Verification items for the finished model (mm, model axes). A direction names the side the tool comes from. Round coordinates to 2 decimals unless told otherwise and drop trailing zeros. Loops run counter-clockwise (first coordinate to the right, second up) from the corner with the lowest first, then second, coordinate; pieces in that order, holes last. Notation, with made-up numbers: (-38.75, 80) -> (-34.75, 80) arc R22 ccw to (-34.75, 103) -> close; hole circle Ø1 at (56, -33). An arc over 180 degrees is marked (long way). Write item = value, one per line.
```python
from build123d import *

# Parameters (mm, degrees)
SKETCH1_W               = 100
SKETCH1_H               = 65
BOSS_EXTRUDE1_DEPTH     = 25
CUT_EXTRUDE1_REACH      = 123.861
SKETCH2_W               = 8.232646472
SKETCH2_H               = 41
SKETCH3_W               = 40
SKETCH3_H               = 25
CUT_EXTRUDE2_DEPTH      = 25
BOSS_EXTRUDE2_DEPTH     = 50
CUT_EXTRUDE3_DEPTH      = 132.244047484
CUT_EXTRUDE3_DEPTH_BACK = 20


with BuildPart() as part:
    # Sketch1 → Boss-Extrude1 (new body)
    with BuildSketch(Plane.XY):
        with Locations((50, 32.5)):
            Rectangle(SKETCH1_W, SKETCH1_H)
    extrude(amount=BOSS_EXTRUDE1_DEPTH)

    # Sketch2 → Cut-Extrude1 (cut, up to next)
    with BuildSketch(Plane(origin=(100, 0, 0), x_dir=(0, 0, -1), z_dir=(1, 0, 0)), mode=Mode.PRIVATE) as cut_extrude1_sk1:
        with Locations((-4.116323236, 32.5)):
            Rectangle(SKETCH2_W, SKETCH2_H)
    cut_extrude1_tool1 = extrude(cut_extrude1_sk1.sketch, amount=-CUT_EXTRUDE1_REACH, mode=Mode.PRIVATE) & part.part
    add(cut_extrude1_tool1.solids().sort_by_distance((100, 32.5, 4.116323))[0], mode=Mode.SUBTRACT)

    # Sketch3 → Cut-Extrude2 (cut)
    with BuildSketch(Plane(origin=(0, 65, 0), x_dir=(1, 0, 0), z_dir=(0, 1, 0))):
        with Locations((50, -12.5)):
            Rectangle(SKETCH3_W, SKETCH3_H)
    extrude(amount=-CUT_EXTRUDE2_DEPTH, mode=Mode.SUBTRACT)

    # Sketch4 → Boss-Extrude2 (add)
    with BuildSketch(Plane.XY.offset(25)):
        Polygon((30, 40), (0, 40), (0, 0), (100, 0), (100, 40), (70, 40), align=None)
    extrude(amount=BOSS_EXTRUDE2_DEPTH)

    # Sketch6 → Cut-Extrude3 (cut, two sides: drawn at the far end of the back side and taken through both)
    with BuildSketch(Plane(origin=(0, 40, 0), x_dir=(1, 0, 0), z_dir=(0, 1, 0)).offset(-CUT_EXTRUDE3_DEPTH_BACK)):
        Polygon((75, -297.132034356), (75, -75), (75, -35), (25, -35), (25, -75), (25, -297.132034356), (25, -741.396103068), (75, -741.396103068), align=None)
    extrude(amount=CUT_EXTRUDE3_DEPTH + CUT_EXTRUDE3_DEPTH_BACK, mode=Mode.SUBTRACT)


solid = part.part
```
(1) Set-up check for faces 1 (the face through (51, 32, 8.233)), 2 (the face through (30, 53, 15)), 3 (the face through (15, 53, 25)), 4 (the face through (50, 30, 35)): record each of +Z, -Z, +X, -X, +Y, -Y from which the full face is reachable in a straight line by a thin tool's end or side.
Filled sheet:
face_1 = -Z, +X, -X
face_2 = +Z, -Z, +Y
face_3 = +Z, +X, -X, +Y
face_4 = +Z, +Y
(2) Go/stop test with flat-tipped pins: pin 1 Ø20.5 at (x, y) = (74.5, 34) entering from -Z; pin 2 Ø7.5 at (x, y) = (8, 51.5) entering from +Z; pin 3 Ø1 at (x, z) = (47.5, 42) entering from +Y. Record where each tip stops, or that it passes through.
Filled sheet:
pin_1 = 8.23
pin_2 = 25
pin_3 = 20
(3) Sectioned sample at B-B, the plane z = 5. Record the cut outline in (x, y).
Filled sheet:
outline = (0, 0) -> (100, 0) -> (100, 12) -> (0, 12) -> close; (0, 53) -> (30, 53) -> (30, 65) -> (0, 65) -> close; (70, 53) -> (100, 53) -> (100, 65) -> (70, 65) -> close
(4) Draft check along Y on faces 5 (the face through (50, 20, 55)), 6 (the face through (51, 12, 4)), 7 (the face through (85, 53, 25)). Enter one of: released by +Y, released by -Y, zero draft, split by the parting line, or undercut.
Filled sheet:
face_5 = released by +Y
face_6 = undercut
face_7 = zero draft
(5) Sectioned sample at C-C, the plane x = 33. Record the cut outline in (y, z).
Filled sheet:
outline = (0, 0) -> (12, 0) -> (12, 8.23) -> (40, 8.23) -> (40, 35) -> (20, 35) -> (20, 75) -> (0, 75) -> close
(6) Sectioned sample at D-D, the plane y = 28. Record the cut outline in (x, z), and give its area (3 significant figures).
Filled sheet:
outline = (0, 8.23) -> (100, 8.23) -> (100, 75) -> (75, 75) -> (75, 35) -> (25, 35) -> (25, 75) -> (0, 75) -> close
area = 4,680 mm2
(7) Sectioned sample at A-A, the plane y = 60.5. Record the cut outline in (x, z), and give its area (3 significant figures).
Filled sheet:
outline = (0, 0) -> (30, 0) -> (30, 25) -> (0, 25) -> close; (70, 0) -> (100, 0) -> (100, 25) -> (70, 25) -> close
area = 1,500 mm2
(8) Material ranges on probe 1 along X at (y, z) = (33, 41); probe 2 along Y at (x, z) = (87.5, 7.5); probe 3 along X at (y, z) = (47.5, 22), recorded low to high. Write a range as from..to.
Filled sheet:
probe_1 = 0..25, 75..100
probe_2 = 0..12, 53..65
probe_3 = 0..30, 70..100
